```python
from build123d import *

# Parameters (mm, degrees)
SKETCH_1_W                       = 77
SKETCH_1_H                       = 32.2
EXTRUDE_1_DEPTH                  = 4
SKETCH_4_R                       = 1.5
CUT_EXTRUDE_3_DEPTH              = 42.92207056
SKETCH_9_R                       = 3
CUT_EXTRUDE_7_DEPTH              = 3
PATTERN_LINEAR_2_COUNT           = 2
PATTERN_LINEAR_2_PITCH           = 38.5
PATTERN_LINEAR_3_COUNT           = 2
PATTERN_LINEAR_3_PITCH           = 24.2
PATTERN_LINEAR_3_COPY_1_SKETCH_R = 1.5
PATTERN_LINEAR_3_COPY_1_DEPTH    = 42.92207056
PATTERN_LINEAR_3_COPY_2_SKETCH_R = 3
PATTERN_LINEAR_3_COPY_2_DEPTH    = 3
SKETCH_12_W                      = 8.2
SKETCH_12_H                      = 8
SKETCH_12_W_2                    = 15.35
CUT_EXTRUDE_13_DEPTH             = 10
PATTERN_LINEAR_5_COUNT           = 2
PATTERN_LINEAR_5_PITCH           = 38.5
CUT_EXTRUDE_14_DEPTH             = 51.349677258


with BuildPart() as part:
    # 草图1 → 凸台-拉伸1 (new body)
    with BuildSketch(Plane.XY):
        Rectangle(SKETCH_1_W, SKETCH_1_H)
    extrude(amount=EXTRUDE_1_DEPTH)

    # 草图4 → 切除-拉伸3 (cut, through all)
    with BuildSketch(Plane(origin=(0, 0, 0), x_dir=(-1, 0, 0), z_dir=(0, 0, -1))):
        with Locations((-27.25, 12.1)):
            Circle(SKETCH_4_R)
        with Locations((-19.25, 12.1)):
            Circle(SKETCH_4_R)
        with Locations((-11.25, 12.1)):
            Circle(SKETCH_4_R)
    cut_extrude_3 = extrude(amount=-CUT_EXTRUDE_3_DEPTH, mode=Mode.SUBTRACT)

    # 草图9 → 切除-拉伸7 (cut)
    with BuildSketch(Plane(origin=(0, 0, 0), x_dir=(-1, 0, 0), z_dir=(0, 0, -1))):
        with Locations((-27.25, 12.1)):
            Circle(SKETCH_9_R)
        with Locations((-19.25, 12.1)):
            Circle(SKETCH_9_R)
        with Locations((-11.25, 12.1)):
            Circle(SKETCH_9_R)
    cut_extrude_7 = extrude(amount=-CUT_EXTRUDE_7_DEPTH, mode=Mode.SUBTRACT)

    # 阵列(线性)2: 切除-拉伸3, 切除-拉伸7 ×2
    with Locations(*[(-i * PATTERN_LINEAR_2_PITCH, 0, 0) for i in range(1, PATTERN_LINEAR_2_COUNT)]):
        add(cut_extrude_3, mode=Mode.SUBTRACT)
        add(cut_extrude_7, mode=Mode.SUBTRACT)

    # 阵列(线性)3: 切除-拉伸3, 切除-拉伸7 ×2
    with Locations(*[(0, -i * PATTERN_LINEAR_3_PITCH, 0) for i in range(1, PATTERN_LINEAR_3_COUNT)]):
        add(cut_extrude_3, mode=Mode.SUBTRACT)
        add(cut_extrude_7, mode=Mode.SUBTRACT)

    # 阵列(线性)3 copy 1 sketch → 阵列(线性)3 copy 1 (cut, through all)
    with BuildSketch(Plane(origin=(-38.5, -24.2, 0), x_dir=(-1, 0, 0), z_dir=(0, 0, -1))):
        with Locations((-27.25, 12.1)):
            Circle(PATTERN_LINEAR_3_COPY_1_SKETCH_R)
        with Locations((-19.25, 12.1)):
            Circle(PATTERN_LINEAR_3_COPY_1_SKETCH_R)
        with Locations((-11.25, 12.1)):
            Circle(PATTERN_LINEAR_3_COPY_1_SKETCH_R)
    extrude(amount=-PATTERN_LINEAR_3_COPY_1_DEPTH, mode=Mode.SUBTRACT)

    # 阵列(线性)3 copy 2 sketch → 阵列(线性)3 copy 2 (cut)
    with BuildSketch(Plane(origin=(-38.5, -24.2, 0), x_dir=(-1, 0, 0), z_dir=(0, 0, -1))):
        with Locations((-27.25, 12.1)):
            Circle(PATTERN_LINEAR_3_COPY_2_SKETCH_R)
        with Locations((-19.25, 12.1)):
            Circle(PATTERN_LINEAR_3_COPY_2_SKETCH_R)
        with Locations((-11.25, 12.1)):
            Circle(PATTERN_LINEAR_3_COPY_2_SKETCH_R)
    extrude(amount=-PATTERN_LINEAR_3_COPY_2_DEPTH, mode=Mode.SUBTRACT)

    # 草图12 → 切除-拉伸13 (cut)
    with BuildSketch(Plane.XY):
        with Locations((-19.25, 12.1)):
            Rectangle(SKETCH_12_W, SKETCH_12_H)
        with Locations((-30.825, -12.1)):
            Rectangle(SKETCH_12_W_2, SKETCH_12_H)
        with Locations((-7.675, -12.1)):
            Rectangle(SKETCH_12_W_2, SKETCH_12_H)
    cut_extrude_13 = extrude(amount=CUT_EXTRUDE_13_DEPTH, mode=Mode.SUBTRACT)

    # 阵列(线性)5: 切除-拉伸13 ×2
    with Locations(*[(i * PATTERN_LINEAR_5_PITCH, 0, 0) for i in range(1, PATTERN_LINEAR_5_COUNT)]):
        add(cut_extrude_13, mode=Mode.SUBTRACT)

    # 草图13 → 切除-拉伸14 (cut, through all)
    with BuildSketch(Plane(origin=(0, 16.1, 0), x_dir=(1, 0, 0), z_dir=(0, 1, 0))):
        Polygon((29.5, 0), (38.5, 0), (38.5, -3), align=None)
        Polygon((-38.5, -1), (-38.5, -4), (-29.5, -4), align=None)
    extrude(amount=-CUT_EXTRUDE_14_DEPTH, mode=Mode.SUBTRACT)


solid = part.part
```
For this review, take the finished solid that the model builds, in its own axes (mm). A direction names the side the tool comes from. Give positions to 0.01 mm unless a question says otherwise; leave off trailing zeros. Write each loop counter-clockwise with the first axis right and the second up, starting at its lowest first coordinate (ties: lowest second). Pieces come first, ordered by that corner, then holes.
Item 1: Machinability: for faces 5 (the face through (29, -8.1, 2)), 6 (the face through (21.631, -13.925, 1.479)), 7 (the face through (19, 8.1, 2)), 8 (the face through (-25.75, 12.17, 3.49)), 9 (the face through (15.35, -12, 2)), which of the approach directions +Z, -Z, +X, -X, +Y, -Y give a long, thin tool a straight path to every point of the face, cutting with its end or side? Answer none if there is none.
Item 2: Take a section at D-D (y = 5). Give the boundary of the cut face in (x, z), and give its area (3 significant figures).
Item 3: Take a section at B-B (z = 1.7). Give the boundary of the cut face in (x, y), and give its area (3 significant figures).
Item 4: Insertion check: P1, Ø1.2, axis at y = -10.5, z = 1, coming from the -X side; P2, Ø3.5, axis at x = 27.25, y = 12.1, coming from the -Z side; P3, Ø1.2, axis at x = 18, z = 2.5, coming from the +Y side. Each pin has a flat end and moves straight along its axis. Give the tip position at first contact, or say it passes through.
Item 5: Take a section at A-A (x = -27.25). Give the boundary of the cut face in (y, z), and give its area (3 significant figures).
Item 6: The part is to be moulded in two halves that separate along X. For faces 1 (the face through (-33.94, 4.17, 2.52)), 2 (the face through (-29, -8.1, 2)), 3 (the face through (23.35, 12, 2)), 4 (the face through (23.15, -12, 2)), say which applies: +X half, -X half, draft (parallel to the pull), parting line (faces both ways), or undercut.
Item 7: Take a section at C-C (y = -12.1). Give the boundary of the cut face in (x, z), and give its area (3 significant figures).
Item 8: Wall thickness on probe 1 along Y at (x, z) = (-11.5, 0.95); probe 2 along Y at (x, z) = (-19.25, 3.7); probe 3 along Z at (x, y) = (27, 9.5): over which ranges is each line inside the solid? List them lowest first.
Established:
1. face 5: +Z, -Z, +X, -Y
1. face 6: -Z
1. face 7: +Z, -Z, +Y
1. face 8: +Z, -Z
1. face 9: +Z, -Z, -Y
2. outline: (-38.5, 0) - (29.5, 0) - (38.5, 3) - (38.5, 4) - (-29.5, 4) - (-38.5, 1) - close
2. area: 281 mm2
3. outline: (-36.4, -8.1) - (-23.15, -8.1) - (-23.15, -16.1) - (-15.35, -16.1) - (-15.35, -8.1) - (15.35, -8.1) - (15.35, -16.1) - (23.15, -16.1) - (23.15, -8.1) - (34.6, -8.1) - (34.6, 16.1) - (23.35, 16.1) - (23.35, 8.1) - (15.15, 8.1) - (15.15, 16.1) - (-15.15, 16.1) - (-15.15, 8.1) - (-23.35, 8.1) - (-23.35, 16.1) - (-36.4, 16.1) - close; hole circle Ø6 at (-27.25, 12.1); hole circle Ø6 at (-19.25, -12.1); hole circle Ø6 at (-11.25, 12.1); hole circle Ø6 at (11.25, 12.1); hole circle Ø6 at (19.25, -12.1); hole circle Ø6 at (27.25, 12.1)
3. area: 1,540 mm2
4. P1: stops at x = -23.15
4. P2: stops at z = 3
4. P3: stops at y = 8.1
5. outline: (-8.1, 0) - (9.1, 0) - (9.1, 3) - (10.6, 3) - (10.6, 4) - (-8.1, 4) - close; (13.6, 3) - (15.1, 3) - (15.1, 0) - (16.1, 0) - (16.1, 4) - (13.6, 4) - close
5. area: 75.8 mm2
6. face 1: -X half
6. face 2: draft
6. face 3: undercut
6. face 4: +X half
7. outline: (-23.15, 0) - (-22.25, 0) - (-22.25, 3) - (-20.75, 3) - (-20.75, 4) - (-23.15, 4) - close; (-17.75, 3) - (-16.25, 3) - (-16.25, 0) - (-15.35, 0) - (-15.35, 4) - (-17.75, 4) - close; (15.35, 0) - (16.25, 0) - (16.25, 3) - (17.75, 3) - (17.75, 4) - (15.35, 4) - close; (20.75, 3) - (22.25, 3) - (22.25, 0) - (23.15, 0) - (23.15, 4) - (20.75, 4) - close
7. area: 20.4 mm2
8. probe 1: y = -8.1 to 9.11, 15.09 to 16.1
8. probe 2: y = -16.1 to -13.6, -10.6 to 8.1
8. probe 3: z = 3 to 4
